Part print with two shaded views. Sizes in mm from the minimum x, y, z corner. Give positions to 0.01 mm unless a question says otherwise; leave off trailing zeros. Order: outer loops, then holes, each group sorted by start corner. A loop starts at its lowest first (then second) coordinate and runs counter-clockwise, first axis right, second up. Notation, with made-up numbers: M 6.25,78 L 10.25,78 A3 cw 10.25,82 Z; hole C -33,80.25 d10. An arc over 180 degrees is marked long. Return JSON: item names as keys, results as strings. Group by question number.
1. Slice it at A-A on y = 15. List the corners of the cut face in (x, z).
2. Slice it at B-B on x = 30. List the corners of the cut face in (y, z).
3. Slice it at D-D on y = 75. List the corners of the cut face in (x, z), then the cut area to 3 significant figures.
4. Wall check: probe 1 along X at (y, z) = (15, 1); probe 2 along Y at (x, z) = (30, 1.15); probe 3 along X at (y, z) = (45, 0.6). Give the ranges that are in metal, low to high. Write a range as [from, to].
5. Slice it at C-C on z = 1.05. List the corners of the cut face in (x, y), then the cut area to 3 significant figures.
6. Pin check, flat tips, straight feed: pin 1 (4 mm diameter, centred on x = 30, y = 45, fed in from -Z); pin 2 (1 mm diameter, centred on x = 9, z = 1.5, fed in from +Y). Stop position of each tip, or through.
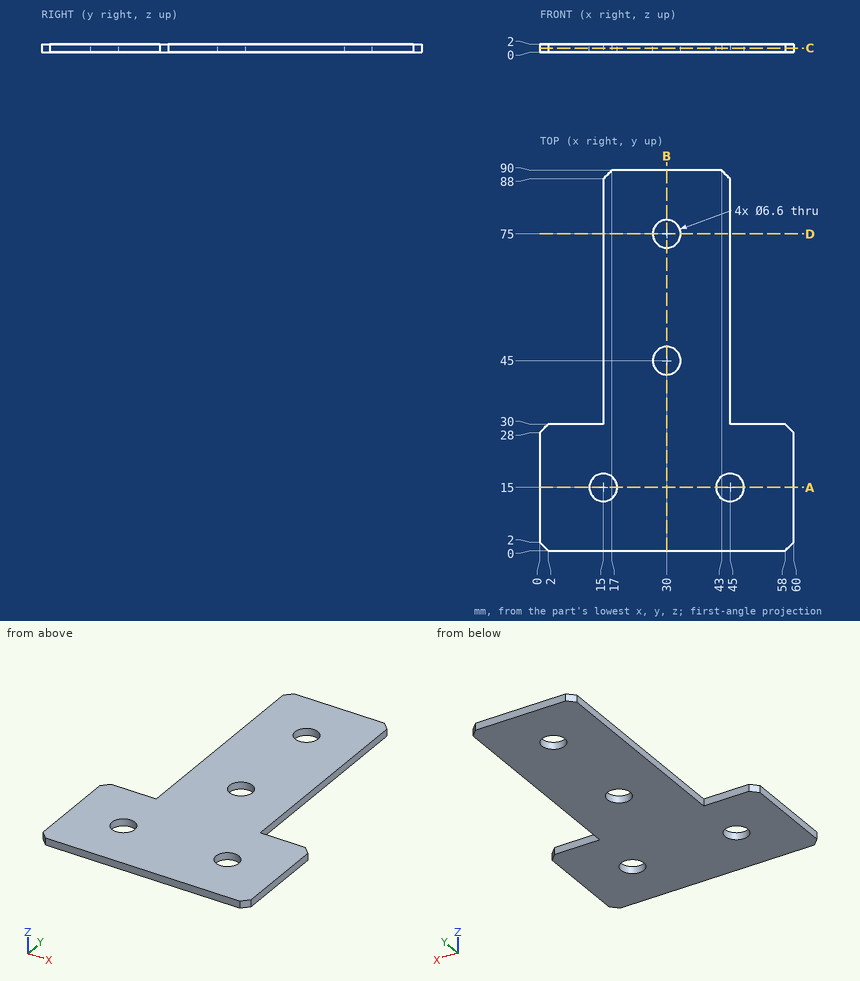
Result:
{
 "1": {"outline": "M 0,0 L 11.7,0 L 11.7,2 L 0,2 Z; M 18.3,0 L 41.7,0 L 41.7,2 L 18.3,2 Z; M 48.3,0 L 60,0 L 60,2 L 48.3,2 Z"},
 "2": {"outline": "M 0,0 L 41.7,0 L 41.7,2 L 0,2 Z; M 48.3,0 L 71.7,0 L 71.7,2 L 48.3,2 Z; M 78.3,0 L 90,0 L 90,2 L 78.3,2 Z"},
 "3": {"outline": "M 15,0 L 26.7,0 L 26.7,2 L 15,2 Z; M 33.3,0 L 45,0 L 45,2 L 33.3,2 Z", "area": "46.8 mm2"},
 "4": {"probe 1": "x = [0, 11.7], [18.3, 41.7], [48.3, 60]", "probe 2": "y = [0, 41.7], [48.3, 71.7], [78.3, 90]", "probe 3": "x = [15, 26.7], [33.3, 45]"},
 "5": {"outline": "M 0,2 L 2,0 L 58,0 L 60,2 L 60,28 L 58,30 L 45,30 L 45,88 L 43,90 L 17,90 L 15,88 L 15,30 L 2,30 L 0,28 Z; hole C 15,15 d6.6; hole C 30,45 d6.6; hole C 30,75 d6.6; hole C 45,15 d6.6", "area": "3,450 mm2"},
 "6": {"pin 1": "passes through", "pin 2": "stops at y = 30"}
}
